The listing builds one solid part. Answer for the finished solid, in the listing's coordinates (mm). A direction names the side the tool comes from. Round coordinates to 2 decimals unless told otherwise and drop trailing zeros. Write each loop counter-clockwise with the first axis right and the second up, starting at its lowest first coordinate (ties: lowest second). Pieces come first, ordered by that corner, then holes. Notation, with made-up numbers: (20.5, 80.25) - (59.5, 80.25) arc R14 cw to (59.5, 100.25) - close; hole circle Ø8 at (71, -35.75). An arc over 180 degrees is marked (long way). Return JSON: item names as keys, results as strings. Group by question number.
(1) Section B-B, the plane x = 113 is taken. Write down the section's boundary in (y, z), then the cut area to 3 significant figures.
(2) Determine the mould class of faces 3 (the flat face through (-2, 0, -2)), 4 (the flat face through (6, 5, -152.64)), 5 (the flat face through (5, 5, 152.64)) for opening direction Z: +Z half, -Z half, draft (parallel to the pull), parting line (faces both ways), or undercut.
(3) Each of these flat-tipped pins is pushed along its axis until it touches: pin 1 (5 mm diameter, centred on x = -89, y = 5.5, fed in from -Z); pin 2 (4 mm diameter, centred on x = -16, z = -58, fed in from -Y). Where does it stop, or does it pass through?
(4) Which of the six approach directions +Z, -Z, +X, -X, +Y, -Y give full straight-line access (tool end or side, diameter ignored) to faces 1 (the flat face through (-84, 5, -121.287)), 2 (the flat face through (-2, 10, -2))?
(5) Find the intervals of material crossed by line 1 along X through (y, z) = (9.25, -134); line 2 along Z through (x, y) = (-70, 8); line 3 along Z through (x, y) = (63.5, 9.5), in increasing order. Write a range as [from, to].
(6) Section A-A, the plane y = 8 is taken. Write down the section's boundary in (x, z), then the cut area to 3 significant figures.
(7) Section C-C, the plane z = 129.5 is taken. Write down the section's boundary in (x, y), then the cut area to 3 significant figures.
```python
from build123d import *

# Parameters (mm, degrees)
SKETCH3_W               = 262.8
SKETCH3_H               = 305.28
BOSS_EXTRUDE3_DEPTH     = 10
CUT_EXTRUDE1_DEPTH      = 202.655472527
CUT_EXTRUDE1_DEPTH_BACK = 202.655472527


with BuildPart() as part:
    # Sketch3 → Boss-Extrude3 (new body)
    with BuildSketch(Plane(origin=(0, 0, 0), x_dir=(1, 0, 0), z_dir=(0, 1, 0))):
        Rectangle(SKETCH3_W, SKETCH3_H)
    extrude(amount=BOSS_EXTRUDE3_DEPTH)

    # Sketch4 → Cut-Extrude1 (cut, two sides: drawn at the far end of the back side and taken through both)
    with BuildSketch(Plane(origin=(0, 10, 0), x_dir=(1, 0, 0), z_dir=(0, 1, 0)).offset(-CUT_EXTRUDE1_DEPTH_BACK)):
        with BuildLine():
            Line((-131.4, -90), (-131.4, -152.64))
            Line((-131.4, -152.64), (-70.92, -152.64))
            ThreePointArc((-70.92, -152.64), (-107.755247271, -127.687824951), (-131.4, -90))
        make_face()
        with BuildLine():
            Line((83.16, -152.64), (131.4, -152.64))
            Line((131.4, -152.64), (131.4, -72.72))
            ThreePointArc((131.4, -72.72), (117.938305095, -119.113391364), (83.16, -152.64))
        make_face()
        with BuildLine():
            Line((-99.372734155, 121.287125755), (-67.345468311, 121.287125755))
            Line((-67.345468311, 121.287125755), (-48.15934209, 152.64))
            Line((-48.15934209, 152.64), (-131.4, 152.64))
            Line((-131.4, 152.64), (-131.4, 83.52))
            ThreePointArc((-131.4, 83.52), (-119.737831056, 106.093689962), (-99.372734155, 121.287125755))
        make_face()
        with BuildLine():
            Line((131.4, 83.52), (131.4, 152.64))
            Line((131.4, 152.64), (62.28, 152.64))
            ThreePointArc((62.28, 152.64), (109.286007047, 130.526007047), (131.4, 83.52))
        make_face()
    extrude(amount=CUT_EXTRUDE1_DEPTH + CUT_EXTRUDE1_DEPTH_BACK, mode=Mode.SUBTRACT)


solid = part.part
```
Working result:
{
 "1": {"outline": "(0, -126.54) - (10, -126.54) - (10, 126.48) - (0, 126.48) - close", "area": "2,530 mm^2"},
 "2": {"face 3": "draft", "face 4": "-Z half", "face 5": "+Z half"},
 "3": {"pin 1": "stops at z = -121.29", "pin 2": "stops at y = 0"},
 "4": {"face 1": "-Z, -X, +Y, -Y", "face 2": "+Z, -Z, +X, -X, +Y"},
 "5": {"line 1": "x = [-59.57, 105.57]", "line 2": "z = [-121.29, 152.64]", "line 3": "z = [-152.52, 152.64]"},
 "6": {"outline": "(-131.4, -83.52) arc R56.58 ccw to (-99.37, -121.29) - (-67.35, -121.29) - (-48.16, -152.64) - (62.28, -152.64) arc R76.66 ccw to (131.4, -83.52) - (131.4, 72.72) arc R93.72 ccw to (83.16, 152.64) - (-70.92, 152.64) arc R107.96 ccw to (-131.4, 90) - close", "area": "73,800 mm^2"},
 "7": {"outline": "(-105.96, 0) - (110.67, 0) - (110.67, 10) - (-105.96, 10) - close", "area": "2,170 mm^2"}
}
